Geometry: final body of the model. Coordinates: model frame, mm. Face numbers are marked on the shaded views. A direction names the side the tool comes from. Give positions to 0.01 mm unless a question says otherwise; leave off trailing zeros. Order: outer loops, then holes, each group sorted by start corner. A loop starts at its lowest first (then second) coordinate and runs counter-clockwise, first axis right, second up. Notation, with made-up numbers: M 48,63 L 84,63 A26 ccw 84,88 Z; hole C 83,57 d4. An arc over 180 degrees is marked long. Use CSV: the item, a comma, the result in double quotes.
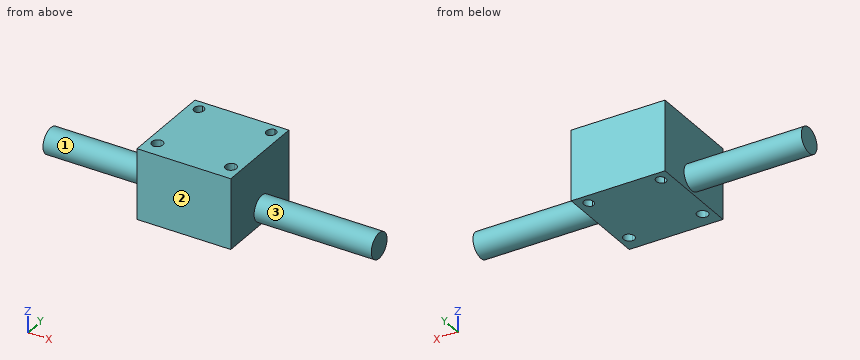
```python
from build123d import *

# Parameters (mm, degrees)
F0_W     = 50.8
F0_H     = 50.8
F0_R     = 3.175
F1_DEPTH = 19.05
F2_R     = 6.872495
F3_DEPTH = 63.5


with BuildPart() as f1:
    # F0 (on Top) → F1 (new body, symmetric)
    with BuildSketch(Plane.XY):
        Rectangle(F0_W, F0_H)
        with Locations((-20.133952, -16.346581)):
            Circle(F0_R, mode=Mode.SUBTRACT)
        with Locations((19.715946, -16.346581)):
            Circle(F0_R, mode=Mode.SUBTRACT)
        with Locations((-20.133952, 19.457644)):
            Circle(F0_R, mode=Mode.SUBTRACT)
        with Locations((19.008903, 19.457644)):
            Circle(F0_R, mode=Mode.SUBTRACT)
    extrude(amount=F1_DEPTH, both=True)

    # F2 (on face) → F3 (join)
    with BuildSketch(Plane(origin=(-25.4, 0, 0), x_dir=(0, -1, 0), z_dir=(-1, 0, 0))):
        with Locations((-1.860697, -10.750698)):
            Circle(F2_R)
    extrude(amount=F3_DEPTH)

    # F4: F1 across plane


with BuildPart() as f1_1:
    add(f1.part)
    add(f1.part.mirror(Plane.YZ))


solid = f1_1.part
```
1. Line query: line 1 (X direction, y = 19.5, z = -10.5); line 2 (Y direction, x = 20, z = -5.5); line 3 (X direction, y = 21.5, z = 16.5). Output: solid intervals per line, ascending.
Answer:
line 1,"-25.4 to -22.18, -16.96 to 16.96, 22.18 to 25.4"
line 2,"-25.4 to -19.51, -13.18 to 16.44, 22.47 to 25.4"
line 3,"-25.4 to -21.44, -17.7 to 17.7, 21.44 to 25.4"
2. Section C-C, the plane x = 35. Return the cut outline in (y, z) (1 decimal), plus the area to 3 significant figures.
Answer:
outline,"C 1.9,-10.8 d13.7"
area,"148 mm2"
3. Section B-B, the plane y = -8. Return the cut outline in (x, z), plus the area to 3 significant figures.
Answer:
outline,"M -25.4,-19.05 L 25.4,-19.05 L 25.4,19.05 L -25.4,19.05 Z"
area,"1,940 mm2"
4. Section A-A, the plane z = 1.5. Return the cut outline in (x, y) (3 decimals).
Answer:
outline,"M -25.4,-25.4 L 25.4,-25.4 L 25.4,25.4 L -25.4,25.4 Z; hole M -19.925,-19.515 A3.175 ccw -19.925,-13.178 A3.175 ccw Z; hole M -19.571,16.333 A3.175 ccw -19.571,22.582 A3.175 ccw Z; hole M 19.571,16.333 A3.175 ccw 19.571,22.582 A3.175 ccw Z; hole M 19.925,-19.515 A3.175 ccw 19.925,-13.178 A3.175 ccw Z"
5. Reachability of the marked faces 1, 2 and 3 from +Z, -Z, +X, -X, +Y, -Y: full face, straight path, thin tool, end or side. Return the list, or none.
Answer:
face 1,"-X"
face 2,"+Z, -Z, +X, -X, -Y"
face 3,"+X"
6. Pin query (flat end, axial travel): pin 1 Ø2 at (x, z) = (40, -7.5) entering from +Y; pin 2 Ø12 at (y, z) = (5, 2.5) entering from +X; pin 3 Ø2 at (y, z) = (-13, 8.5) entering from -X; pin 4 Ø12 at (x, z) = (-42.5, 3) entering from +Y. Return the tip coordinate at first contact, or that it passes through.
Answer:
pin 1,"y = 8.35"
pin 2,"x = 25.4"
pin 3,"x = -25.4"
pin 4,"through"
